```python
from build123d import *

# Parameters (mm, degrees)
SKETCH1_W               = 101.6
SKETCH1_H               = 107.95
BOSS_EXTRUDE1_DEPTH     = 3.175
CUT_EXTRUDE1_DEPTH      = 75.189091179
CUT_EXTRUDE1_DEPTH_BACK = 75.189091179
SKETCH2_W               = 3.429
SKETCH2_H               = 6.604
SKETCH3_W               = 101.6
SKETCH3_H               = 50.8
CUT_EXTRUDE2_DEPTH      = 75.189091179
SKETCH4_W               = 101.6
SKETCH4_H               = 57.15
SKETCH4_R               = 3.429
BOSS_EXTRUDE2_DEPTH     = 3.175


with BuildPart() as part:
    # Sketch1 → Boss-Extrude1 (new body)
    with BuildSketch(Plane(origin=(0, 0, 0), x_dir=(1, 0, 0), z_dir=(0, 1, 0))):
        Rectangle(SKETCH1_W, SKETCH1_H)
    extrude(amount=BOSS_EXTRUDE1_DEPTH)

    # Sketch2 → Cut-Extrude1 (cut, two sides: drawn at the far end of the back side and taken through both)
    with BuildSketch(Plane(origin=(0, 3.175, 0), x_dir=(1, 0, 0), z_dir=(0, 1, 0)).offset(-CUT_EXTRUDE1_DEPTH_BACK)):
        Polygon((22.098, -47.625), (28.194, -47.625), (28.194, -54.229), (34.798, -54.229), (34.798, -47.625), (47.371, -47.625), (47.371, -41.021), (50.8, -41.021), (50.8, -47.625), (50.8, -92.544961432), (-50.8, -92.544961432), (-50.8, -47.625), (-50.8, -41.021), (-47.371, -41.021), (-47.371, -47.625), (-35.306, -47.625), (-35.306, -54.229), (-28.702, -54.229), (-28.702, -47.625), (-22.606, -47.625), (-22.606, -54.229), (-16.002, -54.229), (-16.002, -47.625), (-9.906, -47.625), (-9.906, -54.229), (-3.302, -54.229), (-3.302, -47.625), (2.794, -47.625), (2.794, -54.229), (9.398, -54.229), (9.398, -47.625), (15.494, -47.625), (15.494, -54.229), (22.098, -54.229), align=None)
        with Locations((-49.0855, 31.75)):
            Rectangle(SKETCH2_W, SKETCH2_H)
        with Locations((-49.0855, 19.177)):
            Rectangle(SKETCH2_W, SKETCH2_H)
        with Locations((-49.0855, 6.477)):
            Rectangle(SKETCH2_W, SKETCH2_H)
        with Locations((-49.0855, -6.223)):
            Rectangle(SKETCH2_W, SKETCH2_H)
        with Locations((-49.0855, -18.923)):
            Rectangle(SKETCH2_W, SKETCH2_H)
        with Locations((-49.0855, -31.623)):
            Rectangle(SKETCH2_W, SKETCH2_H)
        with Locations((49.0855, -31.623)):
            Rectangle(SKETCH2_W, SKETCH2_H)
        with Locations((49.0855, -18.923)):
            Rectangle(SKETCH2_W, SKETCH2_H)
        with Locations((49.0855, -6.223)):
            Rectangle(SKETCH2_W, SKETCH2_H)
        with Locations((49.0855, 6.477)):
            Rectangle(SKETCH2_W, SKETCH2_H)
        with Locations((49.0855, 19.177)):
            Rectangle(SKETCH2_W, SKETCH2_H)
        with Locations((49.0855, 31.75)):
            Rectangle(SKETCH2_W, SKETCH2_H)
        with Locations((49.0855, 44.45)):
            Rectangle(SKETCH2_W, SKETCH2_H)
        with Locations((-49.0855, 44.45)):
            Rectangle(SKETCH2_W, SKETCH2_H)
    extrude(amount=CUT_EXTRUDE1_DEPTH + CUT_EXTRUDE1_DEPTH_BACK, mode=Mode.SUBTRACT)

    # Sketch3 → Cut-Extrude2 (cut, through all)
    with BuildSketch(Plane(origin=(0, 3.175, 0), x_dir=(1, 0, 0), z_dir=(0, 1, 0))):
        with Locations((0, 28.575)):
            Rectangle(SKETCH3_W, SKETCH3_H)
    extrude(amount=-CUT_EXTRUDE2_DEPTH, mode=Mode.SUBTRACT)

    # Sketch4 → Boss-Extrude2 (add)
    with BuildSketch(Plane(origin=(0, 3.175, 0), x_dir=(1, 0, 0), z_dir=(0, 1, 0))):
        with Locations((0, 31.75)):
            Rectangle(SKETCH4_W, SKETCH4_H)
        with Locations(Location((-38.1, 15.875, 0), (0, 0, 270))):
            Circle(SKETCH4_R, mode=Mode.SUBTRACT)
        with Locations(Location((-25.4, 15.875, 0), (0, 0, 270))):
            Circle(SKETCH4_R, mode=Mode.SUBTRACT)
        with Locations(Location((-12.7, 15.875, 0), (0, 0, 270))):
            Circle(SKETCH4_R, mode=Mode.SUBTRACT)
        with Locations(Location((0, 15.875, 0), (0, 0, 270))):
            Circle(SKETCH4_R, mode=Mode.SUBTRACT)
        with Locations(Location((12.7, 15.875, 0), (0, 0, 270))):
            Circle(SKETCH4_R, mode=Mode.SUBTRACT)
        with Locations(Location((25.4, 15.875, 0), (0, 0, 270))):
            Circle(SKETCH4_R, mode=Mode.SUBTRACT)
        with Locations(Location((38.1, 15.875, 0), (0, 0, 270))):
            Circle(SKETCH4_R, mode=Mode.SUBTRACT)
        with Locations(Location((-25.4, 28.575, 0), (0, 0, 270))):
            Circle(SKETCH4_R, mode=Mode.SUBTRACT)
        with Locations(Location((-12.7, 28.575, 0), (0, 0, 270))):
            Circle(SKETCH4_R, mode=Mode.SUBTRACT)
        with Locations(Location((0, 28.575, 0), (0, 0, 270))):
            Circle(SKETCH4_R, mode=Mode.SUBTRACT)
        with Locations(Location((12.7, 28.575, 0), (0, 0, 270))):
            Circle(SKETCH4_R, mode=Mode.SUBTRACT)
        with Locations(Location((25.4, 28.575, 0), (0, 0, 270))):
            Circle(SKETCH4_R, mode=Mode.SUBTRACT)
        with Locations(Location((38.1, 28.575, 0), (0, 0, 270))):
            Circle(SKETCH4_R, mode=Mode.SUBTRACT)
        with Locations(Location((-25.4, 41.275, 0), (0, 0, 270))):
            Circle(SKETCH4_R, mode=Mode.SUBTRACT)
        with Locations(Location((-12.7, 41.275, 0), (0, 0, 270))):
            Circle(SKETCH4_R, mode=Mode.SUBTRACT)
        with Locations(Location((0, 41.275, 0), (0, 0, 270))):
            Circle(SKETCH4_R, mode=Mode.SUBTRACT)
        with Locations(Location((12.7, 41.275, 0), (0, 0, 270))):
            Circle(SKETCH4_R, mode=Mode.SUBTRACT)
        with Locations(Location((25.4, 41.275, 0), (0, 0, 270))):
            Circle(SKETCH4_R, mode=Mode.SUBTRACT)
        with Locations(Location((38.1, 41.275, 0), (0, 0, 270))):
            Circle(SKETCH4_R, mode=Mode.SUBTRACT)
        with Locations(Location((-25.4, 53.975, 0), (0, 0, 270))):
            Circle(SKETCH4_R, mode=Mode.SUBTRACT)
        with Locations(Location((-12.7, 53.975, 0), (0, 0, 270))):
            Circle(SKETCH4_R, mode=Mode.SUBTRACT)
        with Locations(Location((0, 53.975, 0), (0, 0, 270))):
            Circle(SKETCH4_R, mode=Mode.SUBTRACT)
        with Locations(Location((12.7, 53.975, 0), (0, 0, 270))):
            Circle(SKETCH4_R, mode=Mode.SUBTRACT)
        with Locations(Location((25.4, 53.975, 0), (0, 0, 270))):
            Circle(SKETCH4_R, mode=Mode.SUBTRACT)
        with Locations(Location((38.1, 53.975, 0), (0, 0, 270))):
            Circle(SKETCH4_R, mode=Mode.SUBTRACT)
        with Locations(Location((-38.1, 28.575, 0), (0, 0, 270))):
            Circle(SKETCH4_R, mode=Mode.SUBTRACT)
        with Locations(Location((-38.1, 41.275, 0), (0, 0, 270))):
            Circle(SKETCH4_R, mode=Mode.SUBTRACT)
        with Locations(Location((-38.1, 53.975, 0), (0, 0, 270))):
            Circle(SKETCH4_R, mode=Mode.SUBTRACT)
    extrude(amount=-BOSS_EXTRUDE2_DEPTH)


solid = part.part
```
Work out the finished part from the listing and answer in its coordinate system (mm). A direction names the side the tool comes from. Give positions to 0.01 mm unless a question says otherwise; leave off trailing zeros. Loops run counter-clockwise (first coordinate to the right, second up) from the corner with the lowest first, then second, coordinate; pieces in that order, holes last. Notation, with made-up numbers: (-37, 4) -> (17, 4) arc R34 ccw to (17, 41) -> close; hole circle Ø4 at (17, 28.5). An arc over 180 degrees is marked (long way). Write item = value, one per line. Start each with the question number.
(1) Find section C-C on z = 8. Give the vertices of the cut face in (x, y) (3 decimals), and give its area (3 significant figures).
(2) Find the intervals of material crossed by probe 1 along Z at (x, y) = (-12.5, 1.6) (3 decimals); probe 2 along Z at (x, y) = (-10, 3) (3 decimals); probe 3 along Z at (x, y) = (-46, 1.9) (3 decimals), in increasing order. Write a range as from..to.
(3) Find section B-B on y = 0.5. Give the number of separate pieces and of enclosed holes in the cut face, and give its area (3 significant figures).
(4) The mould has two halves that part along Z. Classify faces 6 (the flat face through (0, 2, 47.625)), 7 (the cylindrical face through (-39.4, 1.6, -38.1)), 8 (the flat face through (-50.8, 2, -28)): +Z half, -Z half, draft (parallel to the pull), parting line (faces both ways), or undercut.
(5) Given pin 1 Ø1.6 at (y, z) = (1.5, 51.5) entering from +X; pin 2 Ø1 at (y, z) = (2, 5) entering from -X; pin 3 Ø1.6 at (y, z) = (1, 50.5) entering from -X, each flat-ended and moving along its own axis, determine where each tip first touches the part or whether it passes through.
(6) Which of the six approach directions +Z, -Z, +X, -X, +Y, -Y give full straight-line access (tool end or side, diameter ignored) to faces 1 (the flat face through (-49, 2, 9.525)), 2 (the flat face through (34.798, 2, 51)), 3 (the flat face through (49, 2, 28.321)), 4 (the flat face through (-47.371, 2, 44)), 5 (the flat face through (22.098, 2, 51))?
(7) Find section A-A on x = 38.1. Give the vertices of the cut face in (y, z) (3 decimals), and give its area (3 significant figures).
From the geometry:
q1.outline = (-47.371, 0) -> (47.371, 0) -> (47.371, 3.175) -> (-47.371, 3.175) -> close
q1.area = 301 mm^2
q2.probe_1 = -60.325..-57.398, -50.552..-44.698, -37.852..-31.998, -25.152..-19.298, -12.452..47.625
q2.probe_2 = -60.325..-56.089, -51.861..-43.389, -39.161..-30.689, -26.461..-17.989, -13.761..47.625
q2.probe_3 = -60.325..47.625
q3.separate_pieces = 1
q3.enclosed_holes = 28
q3.area = 10,000 mm^2
q4.face_6 = +Z half
q4.face_7 = undercut
q4.face_8 = draft
q5.pin_1 = 34.8
q5.pin_2 = -47.37
q5.pin_3 = -35.31
q6.face_1 = -X, +Y, -Y
q6.face_2 = +Z, +X, +Y, -Y
q6.face_3 = +X, +Y, -Y
q6.face_4 = +Z, -X, +Y, -Y
q6.face_5 = +Z, +Y, -Y
q7.outline = (0, -60.325) -> (3.175, -60.325) -> (3.175, -57.404) -> (0, -57.404) -> close; (0, -50.546) -> (3.175, -50.546) -> (3.175, -44.704) -> (0, -44.704) -> close; (0, -37.846) -> (3.175, -37.846) -> (3.175, -32.004) -> (0, -32.004) -> close; (0, -25.146) -> (3.175, -25.146) -> (3.175, -19.304) -> (0, -19.304) -> close; (0, -12.446) -> (3.175, -12.446) -> (3.175, 47.625) -> (0, 47.625) -> close
q7.area = 256 mm^2
